Part model, mm, in its own coordinate system. A direction names the side the tool comes from. Give positions to 0.01 mm unless a question says otherwise; leave off trailing zeros. Order: outer loops, then holes, each group sorted by start corner. A loop starts at its lowest first (then second) coordinate and runs counter-clockwise, first axis right, second up.
Autodesk Inventor part; units mm, degrees
ref_plane "YZ Plane" through (0, 0, 0) normal (1, 0, 0) x (0, 1, 0)
ref_plane "XZ Plane" through (0, 0, 0) normal (0, 1, 0) x (-1, 0, 0)
ref_plane "XY Plane" through (0, 0, 0) normal (0, 0, 1) x (1, 0, 0)
sketch "Skizze1" plane through (0, 0, 0) normal (0, 0, 1) x (1, 0, 0)
  line L0 (-10, -4.05) -> (10, -4.05)
  line L1 (10, -4.05) -> (10, 4.05)
  line L2 (10, 4.05) -> (-10, 4.05)
  line L3 (-10, 4.05) -> (-10, -4.05)
  line L4 (-10, -4.05) -> (10, 4.05) construction
  line L5 (10, -4.05) -> (-10, 4.05) construction
  point P0 (0, 0)
  dimension "d0" = 20
  dimension "d1" = 8.1
extrude "Extrusion1" add sketch "Skizze1" along normal blind 10
sketch "Skizze2" plane through (0, 0, 10) normal (0, 0, 1) x (1, 0, 0)
  circle A0 centre (-7.46, 0) radius 1.9
  circle A1 centre (-2.46, 0) radius 1.9
  line L0 (-10, 4.05) -> (-10, -4.05)
  circle A2 centre (2.54, 0) radius 1.9
  circle A3 centre (7.54, 0) radius 1.9
  point P0 (0, 0)
  point P1 (-10, 0)
  dimension "d6" = 3.8
  dimension "d7" = 3.8
  dimension "d56" = 2.54
  dimension "d57" = 5
  dimension "d58" = 3.8
  dimension "d59" = 3.8
  dimension "d60" = 5
  dimension "d61" = 5
extrude "Extrusion2" cut sketch "Skizze2" against normal blind 0.45
chamfer "Fasen1" distance 1.55 distance2 4.59 1 edges at (0, -4.05, 10) measured on face at (-0.7437, -3.3287, 10)
chamfer "Fasen2" distance 1.55 distance2 5.5 1 edges at (0, 4.05, 10) measured on face at (0.7703, 3.3287, 10)
sketch "Skizze3" plane through (0, 0, 0) normal (0, 0, -1) x (-1, 0, 0)
  line L0 (2.81, 0.25) -> (2.11, 0.25)
  line L1 (2.11, 0.25) -> (2.11, -0.25)
  line L2 (2.11, -0.25) -> (2.81, -0.25)
  line L3 (2.81, -0.25) -> (2.81, 0.25)
  line L4 (2.81, 0.25) -> (2.11, -0.25) construction
  line L5 (2.11, 0.25) -> (2.81, -0.25) construction
  line L6 (7.11, 0.25) -> (7.81, 0.25)
  line L7 (7.81, 0.25) -> (7.81, -0.25)
  line L8 (7.81, -0.25) -> (7.11, -0.25)
  line L9 (7.11, -0.25) -> (7.11, 0.25)
  line L10 (7.11, 0.25) -> (7.81, -0.25) construction
  line L11 (7.81, 0.25) -> (7.11, -0.25) construction
  line L12 (10, 4.05) -> (10, -4.05)
  line L13 (-2.19, -0.25) -> (-2.89, -0.25)
  line L14 (-2.89, -0.25) -> (-2.89, 0.25)
  line L15 (-2.89, 0.25) -> (-2.19, 0.25)
  line L16 (-2.19, 0.25) -> (-2.19, -0.25)
  line L17 (-2.19, -0.25) -> (-2.89, 0.25) construction
  line L18 (-2.89, -0.25) -> (-2.19, 0.25) construction
  line L19 (-7.19, -0.25) -> (-7.89, -0.25)
  line L20 (-7.89, -0.25) -> (-7.89, 0.25)
  line L21 (-7.89, 0.25) -> (-7.19, 0.25)
  line L22 (-7.19, 0.25) -> (-7.19, -0.25)
  line L23 (-7.19, -0.25) -> (-7.89, 0.25) construction
  line L24 (-7.89, -0.25) -> (-7.19, 0.25) construction
  point P0 (2.46, 0)
  point P1 (7.46, 0)
  point P2 (-2.54, 0)
  point P3 (-7.54, 0)
  dimension "d18" = 0.7
  dimension "d19" = 0.5
  dimension "d20" = 0.7
  dimension "d21" = 0.5
  dimension "d43" = 2.54
  dimension "d45" = 5
  dimension "d48" = 0.7
  dimension "d49" = 0.5
  dimension "d50" = 5
  dimension "d51" = 0.7
  dimension "d52" = 0.5
  dimension "d53" = 5
extrude "Extrusion3" add sketch "Skizze3" along normal blind 3.5
fillet "Rundung1" radius 0.25 16 edges at (-7.81, 0, -3.5) (-7.11, 0, -3.5) (-7.46, -0.25, -3.5) (-7.46, 0.25, -3.5) (-2.46, -0.25, -3.5) (-2.81, 0, -3.5) (-2.46, 0.25, -3.5) (-2.11, 0, -3.5) (2.54, -0.25, -3.5) (2.19, 0, -3.5) (2.54, 0.25, -3.5) (2.89, 0, -3.5) (7.54, -0.25, -3.5) (7.89, 0, -3.5) (7.54, 0.25, -3.5) (7.19, 0, -3.5)
sketch "Skizze5" plane through (-10, -4.05, 0) normal (0, -1, 0) x (1, 0, 0)
  line L0 (4.04, 1.205) -> (1.04, 1.205)
  line L1 (1.04, 1.205) -> (1.04, 4.205)
  line L2 (1.04, 4.205) -> (4.04, 4.205)
  line L3 (4.04, 4.205) -> (4.04, 1.205)
  line L4 (4.04, 1.205) -> (1.04, 4.205) construction
  line L5 (1.04, 1.205) -> (4.04, 4.205) construction
  line L6 (6.04, 1.205) -> (9.04, 1.205)
  line L7 (9.04, 1.205) -> (9.04, 4.205)
  line L8 (9.04, 4.205) -> (6.04, 4.205)
  line L9 (6.04, 4.205) -> (6.04, 1.205)
  line L10 (6.04, 1.205) -> (9.04, 4.205) construction
  line L11 (9.04, 1.205) -> (6.04, 4.205) construction
  line L12 (11.04, 1.205) -> (14.04, 1.205)
  line L13 (14.04, 1.205) -> (14.04, 4.205)
  line L14 (14.04, 4.205) -> (11.04, 4.205)
  line L15 (11.04, 4.205) -> (11.04, 1.205)
  line L16 (11.04, 1.205) -> (14.04, 4.205) construction
  line L17 (14.04, 1.205) -> (11.04, 4.205) construction
  line L18 (0, 0) -> (0, 5.41)
  line L19 (16.04, 1.205) -> (19.04, 1.205)
  line L20 (19.04, 1.205) -> (19.04, 4.205)
  line L21 (19.04, 4.205) -> (16.04, 4.205)
  line L22 (16.04, 4.205) -> (16.04, 1.205)
  line L23 (16.04, 1.205) -> (19.04, 4.205) construction
  line L24 (19.04, 1.205) -> (16.04, 4.205) construction
  point P0 (10, 0)
  point P1 (2.54, 2.705)
  point P2 (7.54, 2.705)
  point P3 (12.54, 2.705)
  point P4 (17.54, 2.705)
  dimension "d27" = 3
  dimension "d28" = 3
  dimension "d29" = 3
  dimension "d30" = 3
  dimension "d31" = 3
  dimension "d32" = 3
  dimension "d33" = 2.54
  dimension "d34" = 5
  dimension "d35" = 5
  dimension "d40" = 3
  dimension "d41" = 3
  dimension "d42" = 5
extrude "Extrusion5" cut sketch "Skizze5" against normal blind 2
properties part number "Schraubklemme_1x3"
Item 1: Band-saw the part on C-C on z = 7.75. List the corners of the cut face in (x, y), plus the area to 3 significant figures.
Item 2: Band-saw the part on D-D on x = 1.5. List the corners of the cut face in (y, z) (3 decimals), plus the area to 3 significant figures.
Item 3: Pull direction Y, two halves, no side cores. Call faces 4 (the face through (10, 0, 5)), 5 (the face through (-2, 0, 9.55)), 6 (the face through (0.14, 3.286, 7.211)): released by +Y, released by -Y, zero draft, split by the parting line, or undercut.
Item 4: Which spindle directions (+Z, -Z, +X, -X, +Y, -Y) get a long thin tool onto all of the face, cutting with end or side? Do faces 1 (the face through (0, 0, 10)), 2 (the face through (5.64, 0.08, 9.78)), 3 (the face through (-7, -3, 4.205)). Say none if no direction does.
Item 5: Drop flat-ended pins along their axis: P1, Ø0.6, axis at y = 0, z = -2, coming from the +X side; P2, Ø0.6, axis at y = 0, z = -1.5, coming from the -X side; P3, Ø1.1, axis at x = 2, y = -0.5, coming from the +Z side. Give the stop position or say it passes through.
Item 6: Band-saw the part on A-A on y = 1. List the corners of the cut face in (x, z).
Item 7: Drill centre lines: probe 1 along Z at (x, y) = (-1.75, 1.5); probe 2 along Z at (x, y) = (-0.5, 1.5); probe 3 along Y at (x, z) = (7.54, 9.9). Where is each one in solid material? Low to high.
Item 8: Band-saw the part on B-B on x = -3.75. List the corners of the cut face in (y, z) (3 decimals).
Working result:
1. outline: (-10, -3.26) - (10, -3.26) - (10, 3.13) - (-10, 3.13) - close
1. area: 128 mm2
2. outline: (-4.05, 0) - (4.05, 0) - (4.05, 4.5) - (2.5, 10) - (1.59, 10) - (1.59, 9.55) - (-1.59, 9.55) - (-1.59, 10) - (-2.5, 10) - (-4.05, 5.41) - (-4.05, 4.205) - (-2.05, 4.205) - (-2.05, 1.205) - (-4.05, 1.205) - close
2. area: 65.7 mm2
3. face 4: zero draft
3. face 5: undercut
3. face 6: released by +Y
4. face 1: +Z, +X, -X, +Y, -Y
4. face 2: +Z
4. face 3: -Y
5. P1: stops at x = 7.89
5. P2: stops at x = -7.81
5. P3: stops at z = 9.55
6. outline: (-10, 0) - (10, 0) - (10, 10) - (9.16, 10) - (9.16, 9.55) - (5.92, 9.55) - (5.92, 10) - (4.16, 10) - (4.16, 9.55) - (0.92, 9.55) - (0.92, 10) - (-0.84, 10) - (-0.84, 9.55) - (-4.08, 9.55) - (-4.08, 10) - (-5.84, 10) - (-5.84, 9.55) - (-9.08, 9.55) - (-9.08, 10) - (-10, 10) - close
7. probe 1: z = 0 to 9.55
7. probe 2: z = 0 to 10
7. probe 3: y = -2.53 to -1.9, 1.9 to 2.53
8. outline: (-4.05, 0) - (4.05, 0) - (4.05, 4.5) - (2.5, 10) - (1.395, 10) - (1.395, 9.55) - (-1.395, 9.55) - (-1.395, 10) - (-2.5, 10) - (-4.05, 5.41) - (-4.05, 4.205) - (-2.05, 4.205) - (-2.05, 1.205) - (-4.05, 1.205) - close
